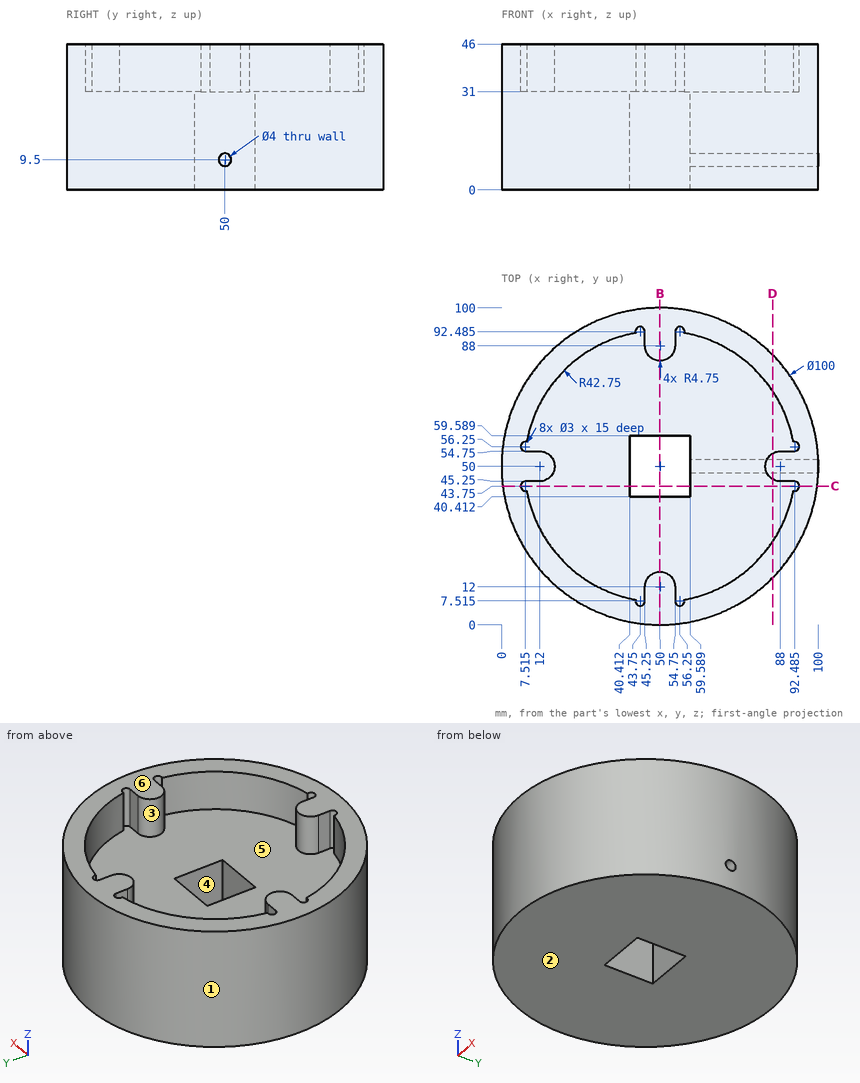
Design review of the part shown in the three views and the two pictorial views. Dimensions are in mm from the part's minimum x, y and z. A direction names the side the tool comes from. Round coordinates to 2 decimals unless told otherwise and drop trailing zeros. Order: outer loops, then holes, each group sorted by start corner. A loop starts at its lowest first (then second) coordinate and runs counter-clockwise, first axis right, second up. Notation, with made-up numbers: M 39.25,-34.5 L 63.25,-34.5 A17 ccw 63.25,-24.5 Z; hole C 9.5,37 d3. An arc over 180 degrees is marked long. Put each result on its own line as item: value.
Q1. Consider section C-C (y = 43.75). State the section outline as (x, z) points (1 decimal), and give its area (3 significant figures).
Reported:
outline: M 0.4,0 L 40.4,0 L 40.4,31 L 6,31 L 6,46 L 0.4,46 Z; M 59.6,0 L 99.6,0 L 99.6,46 L 94,46 L 94,31 L 59.6,31 Z
area: 2,650 mm²
Q2. Consider section B-B (x = 50). State the section outline as (y, z) points, and give its area (3 significant figures).
Reported:
outline: M 0,0 L 40.41,0 L 40.41,31 L 16.75,31 L 16.75,46 L 0,46 Z; M 59.59,0 L 100,0 L 100,46 L 83.25,46 L 83.25,31 L 59.59,31 Z
area: 3,010 mm²
Q3. To check wall thickness, follow line 1 (X direction, y = 43, z = 37) (1 decimal); line 2 (X direction, y = 56.5, z = 36) (1 decimal); line 3 (Z direction, x = 80.5, y = 31). State the ranges of each line that lie inside material, in increasing order.
Reported:
line 1: 0.5 to 6.2, 93.8 to 99.5
line 2: 0.4 to 6, 94 to 99.6
line 3: 0 to 31
Q4. Draft analysis for pull direction X (two halves, no side actions). For the marked faces 1, 2 and 3, state which applies: released by +X, released by -X, zero draft, split by the parting line, or undercut.
Reported:
face 1: split by the parting line
face 2: zero draft
face 3: undercut
Q5. Insertion check: pin 1 Ø1 at (x, y) = (41, 37) entering from +Z; pin 2 Ø6 at (y, z) = (80, 5) entering from -X; pin 3 Ø2 at (y, z) = (76, 40.5) entering from +X. Each pin has a flat end and moves straight along its axis. Give the tip position at first contact, or say it passes through.
Reported:
pin 1: z = 31
pin 2: x = 7.92
pin 3: x = 93.3
Q6. Consider section D-D (x = 85.5). State the section outline as (y, z) points.
Reported:
outline: M 14.79,0 L 85.21,0 L 85.21,46 L 73.82,46 L 73.82,31 L 54.04,31 L 54.04,46 L 45.96,46 L 45.96,31 L 26.18,31 L 26.18,46 L 14.79,46 Z; hole C 50,9.5 d4
Q7. Machinability: for the marked faces 4, 5 and 6, which of the approach directions +Z, -Z, +X, -X, +Y, -Y give a long, thin tool a straight path to every point of the face, cutting with its end or side? Answer none if there is none.
Reported:
face 4: +Z, -Z
face 5: +Z
face 6: +Z, +X, -X, +Y, -Y
